from build123d import *

# Parameters (mm, degrees)
SKETCH1_W                                           = 70
SKETCH1_H                                           = 70
BOSS_EXTRUDE1_DEPTH                                 = 65
FILLET1_R                                           = 15
SKETCH2_R                                           = 27.5
CUT_EXTRUDE1_DEPTH                                  = 65
CUT_EXTRUDE2_DEPTH                                  = 71
CUT_EXTRUDE3_DEPTH                                  = 71
CUT_EXTRUDE4_START                                  = -10
SKETCH10_W                                          = 15
SKETCH10_H                                          = 15
CUT_EXTRUDE4_DEPTH                                  = 45
CBORE_FOR_M3_HEX_SOCKET_HEAD_CAP_SCREW1_D           = 3.4
CBORE_FOR_M3_HEX_SOCKET_HEAD_CAP_SCREW1_DEPTH       = 10
CBORE_FOR_M3_HEX_SOCKET_HEAD_CAP_SCREW1_CBORE_D     = 6.5
CBORE_FOR_M3_HEX_SOCKET_HEAD_CAP_SCREW1_CBORE_DEPTH = 3.4
FILLET2_R                                           = 3
CBORE_FOR_M3_HEX_SOCKET_HEAD_CAP_SCREW2_D           = 3.4
CBORE_FOR_M3_HEX_SOCKET_HEAD_CAP_SCREW2_DEPTH       = 10
CBORE_FOR_M3_HEX_SOCKET_HEAD_CAP_SCREW2_CBORE_D     = 6.5
CBORE_FOR_M3_HEX_SOCKET_HEAD_CAP_SCREW2_CBORE_DEPTH = 3.4
FILLET3_R                                           = 5


with BuildPart() as part:
    # Sketch1 → Boss-Extrude1 (new body)
    with BuildSketch(Plane(origin=(0, 0, 0), x_dir=(1, 0, 0), z_dir=(0, 1, 0))):
        Rectangle(SKETCH1_W, SKETCH1_H)
    extrude(amount=BOSS_EXTRUDE1_DEPTH)

    # Fillet1
    fillet1_edges = [part.edges().sort_by_distance(p)[0] for p in [
        (-35, 32.5, -35),
        (35, 32.5, -35),
        (35, 32.5, 35),
        (-35, 32.5, 35),
    ]]
    fillet(fillet1_edges, radius=FILLET1_R)

    # Sketch2 → Cut-Extrude1 (cut)
    with BuildSketch(Plane(origin=(0, 65, 0), x_dir=(1, 0, 0), z_dir=(0, 1, 0))):
        Circle(SKETCH2_R)
    extrude(amount=-CUT_EXTRUDE1_DEPTH, mode=Mode.SUBTRACT)

    # Sketch3 → Cut-Extrude2 (cut, through all)
    with BuildSketch(Plane(origin=(0, 0, -35), x_dir=(-1, 0, 0), z_dir=(0, 0, -1))):
        Polygon((-10, 10), (-10, 45), (-4, 55), (4, 55), (10, 45), (10, 10), align=None)
    extrude(amount=-CUT_EXTRUDE2_DEPTH, mode=Mode.SUBTRACT)

    # Sketch4 → Cut-Extrude3 (cut, through all)
    with BuildSketch(Plane(origin=(35, 0, 0), x_dir=(0, 0, -1), z_dir=(1, 0, 0))):
        Polygon((-10, 10), (-10, 45), (-4, 55), (4, 55), (10, 45), (10, 10), align=None)
    extrude(amount=-CUT_EXTRUDE3_DEPTH, mode=Mode.SUBTRACT)

    # Sketch10 → Cut-Extrude4 (cut)
    with BuildSketch(Plane(origin=(0, 65, 0), x_dir=(1, 0, 0), z_dir=(0, 1, 0)).offset(CUT_EXTRUDE4_START)):
        with Locations((-27.5, 27.5)):
            Rectangle(SKETCH10_W, SKETCH10_H)
        with Locations((-27.5, -27.5)):
            Rectangle(SKETCH10_W, SKETCH10_H)
        with Locations((27.5, -27.5)):
            Rectangle(SKETCH10_W, SKETCH10_H)
        with Locations((27.5, 27.5)):
            Rectangle(SKETCH10_W, SKETCH10_H)
    extrude(amount=-CUT_EXTRUDE4_DEPTH, mode=Mode.SUBTRACT)

    # CBORE for M3 Hex Socket Head Cap Screw1
    with Locations(Plane(origin=(0, 55, 0), x_dir=(-1, 0, 0), z_dir=(0, -1, 0))):
        with Locations((26, -26), (-26, -26), (-26, 26), (26, 26)):
            CounterBoreHole(CBORE_FOR_M3_HEX_SOCKET_HEAD_CAP_SCREW1_D / 2, CBORE_FOR_M3_HEX_SOCKET_HEAD_CAP_SCREW1_CBORE_D / 2, CBORE_FOR_M3_HEX_SOCKET_HEAD_CAP_SCREW1_CBORE_DEPTH, depth=CBORE_FOR_M3_HEX_SOCKET_HEAD_CAP_SCREW1_DEPTH)

    # Fillet2
    fillet2_edges = [part.edges().sort_by_distance(p)[0] for p in [
        (20, 32.5, -20),
        (20, 32.5, 20),
        (-20, 32.5, 20),
        (-20, 32.5, -20),
    ]]
    fillet(fillet2_edges, radius=FILLET2_R)

    # CBORE for M3 Hex Socket Head Cap Screw2
    with Locations(Plane(origin=(0, 10, 0), x_dir=(1, 0, 0), z_dir=(0, 1, 0))):
        with Locations((26, -26), (26, 26), (-26, 26), (-26, -26)):
            CounterBoreHole(CBORE_FOR_M3_HEX_SOCKET_HEAD_CAP_SCREW2_D / 2, CBORE_FOR_M3_HEX_SOCKET_HEAD_CAP_SCREW2_CBORE_D / 2, CBORE_FOR_M3_HEX_SOCKET_HEAD_CAP_SCREW2_CBORE_DEPTH, depth=CBORE_FOR_M3_HEX_SOCKET_HEAD_CAP_SCREW2_DEPTH)

    # Fillet3
    fillet3_edges = [part.edges().sort_by_distance(p)[0] for p in [
        (35, 32.5, -20),
        (20, 32.5, -35),
        (35, 32.5, 20),
        (20, 32.5, 35),
        (-35, 32.5, 20),
        (-20, 32.5, 35),
        (-20, 32.5, -35),
        (-35, 32.5, -20),
    ]]
    fillet(fillet3_edges, radius=FILLET3_R)


solid = part.part
CAD build for the part. Positions are in the model's coordinates, mm. A direction names the side the tool comes from. Give positions to 0.01 mm unless a question says otherwise; leave off trailing zeros. Order: outer loops, then holes, each group sorted by start corner. A loop starts at its lowest first (then second) coordinate and runs counter-clockwise, first axis right, second up. Notation, with made-up numbers: (74, 11.5) -> (93, 11.5) arc R22 cw to (93, 31.5) -> close; hole circle Ø11 at (-37.75, 25.25). An arc over 180 degrees is marked (long way). Return JSON: item names as keys, results as strings.
Q1. Saw through at C-C (x = 1). Write the cut outline in (y, z).
Working result:
{"outline": "(0, -35) -> (10, -35) -> (10, -27.48) -> (0, -27.48) -> close; (0, 27.48) -> (10, 27.48) -> (10, 35) -> (0, 35) -> close; (55, -35) -> (65, -35) -> (65, -27.48) -> (55, -27.48) -> close; (55, 27.48) -> (65, 27.48) -> (65, 35) -> (55, 35) -> close"}
Q2. Which spindle directions (+Z, -Z, +X, -X, +Y, -Y) get a long thin tool onto all of the face, cutting with end or side? Do faces 5 (the face through (-19, 32, 33)), 6 (the face through (-27.4, 58.4, -24.6)), 7 (the face through (20.86, 32.18, 20.9)). Say none if no direction does.
Working result:
{"face 5": "+Z, -X", "face 6": "none", "face 7": "+Z, +X"}
Q3. Flat gauge pins, fed straight in: pin 1 (2.5 mm diameter, centred on x = 26, z = -26, fed in from -Y); pin 2 (7.5 mm diameter, centred on y = 28.5, z = -32, fed in from +X); pin 3 (4 mm diameter, centred on x = -24, y = 57, fed in from -Z); pin 4 (10.5 mm diameter, centred on y = 30, z = 30.5, fed in from -X). Where does each tip first touch, or does it go through?
Working result:
{"pin 1": "through", "pin 2": "x = 20", "pin 3": "z = -34.87", "pin 4": "x = -20"}
Q4. Saw through at A-A (z = 11.5). Write the cut outline in (x, y), then the cut area to 3 significant figures.
Working result:
{"outline": "(-35, 0) -> (-24.98, 0) -> (-24.98, 65) -> (-35, 65) -> close; (24.98, 0) -> (35, 0) -> (35, 65) -> (24.98, 65) -> close", "area": "1,300 mm²"}
Q5. Drill centre lines: line 1 (Y direction, x = -23.5, z = 31); line 2 (Z direction, x = -28.5, y = 44). Where is each one in solid material? Low to high.
Working result:
{"line 1": "0 to 10, 55 to 65", "line 2": "-20 to -10, 10 to 20"}
Q6. Saw through at B-B (z = 0). Write the cut outline in (x, y), then the cut area to 3 significant figures.
Working result:
{"outline": "(-35, 0) -> (-27.5, 0) -> (-27.5, 10) -> (-35, 10) -> close; (-35, 55) -> (-27.5, 55) -> (-27.5, 65) -> (-35, 65) -> close; (27.5, 0) -> (35, 0) -> (35, 10) -> (27.5, 10) -> close; (27.5, 55) -> (35, 55) -> (35, 65) -> (27.5, 65) -> close", "area": "300 mm²"}
Q7. Saw through at D-D (x = 14). Write the cut outline in (y, z).
Working result:
{"outline": "(0, -35) -> (65, -35) -> (65, -23.67) -> (0, -23.67) -> close; (0, 23.67) -> (65, 23.67) -> (65, 35) -> (0, 35) -> close"}
Q8. Mould opens along X. For faces 1 (the face through (27.4, 6.6, 27.4)), 2 (the face through (-18, 32, -34)), 3 (the face through (20, 33, 27)), 4 (the face through (-30, 28, -10)) say: pulls with the +X half, pulls with the -X half, needs draft (parallel to the pull), parting line crosses it, or undercut.
Working result:
{"face 1": "undercut", "face 2": "pulls with the -X half", "face 3": "pulls with the +X half", "face 4": "needs draft"}
